Geometry: final body of the model. Coordinates: model frame, mm. Face numbers are marked on the shaded views. Coordinates: 2 decimals unless noted, no trailing zeros. Loops run counter-clockwise (first coordinate to the right, second up) from the corner with the lowest first, then second, coordinate; pieces in that order, holes last. Notation, with made-up numbers: (59, 29.25) -> (64, 29.25) arc R31 ccw to (64, 54.25) -> close; hole circle Ø3 at (-28.5, -8.75). An arc over 180 degrees is marked (long way). One line per item, written item: value. Start each with the question number.
from build123d import *

# Parameters (mm, degrees)
SKETCH1_W           = 118
SKETCH1_H           = 70
BOSS_EXTRUDE1_DEPTH = 36
FILLET1_R           = 2
SKETCH2_W           = 15
SKETCH2_H           = 8
CUT_EXTRUDE1_DEPTH  = 10


with BuildPart() as part:
    # Sketch1 → Boss-Extrude1 (new body)
    with BuildSketch(Plane(origin=(0, 0, 0), x_dir=(1, 0, 0), z_dir=(0, 1, 0))):
        Rectangle(SKETCH1_W, SKETCH1_H)
    extrude(amount=BOSS_EXTRUDE1_DEPTH)

    # Fillet1
    fillet1_edges = [part.edges().sort_by_distance(p)[0] for p in [
        (-59, 36, 0),
        (0, 36, 35),
        (59, 36, 0),
        (0, 0, 35),
        (-59, 0, 0),
        (0, 0, -35),
        (59, 0, 0),
        (59, 18, 35),
        (-59, 18, 35),
        (-59, 18, -35),
        (59, 18, -35),
        (0, 36, -35),
    ]]
    fillet(fillet1_edges, radius=FILLET1_R)

    # Sketch2 → Cut-Extrude1 (cut)
    with BuildSketch(Plane.ZY.offset(59)):
        with Locations((-22.5, 18)):
            Rectangle(SKETCH2_W, SKETCH2_H)
        with Locations((23.5, 18)):
            Rectangle(SKETCH2_W, SKETCH2_H)
        with BuildLine():
            Line((-3, 20.5), (2, 20.5))
            ThreePointArc((2, 20.5), (4.5, 18), (2, 15.5))
            Line((2, 15.5), (-3, 15.5))
            ThreePointArc((-3, 15.5), (-5.5, 18), (-3, 20.5))
        make_face()
    extrude(amount=-CUT_EXTRUDE1_DEPTH, mode=Mode.SUBTRACT)


solid = part.part
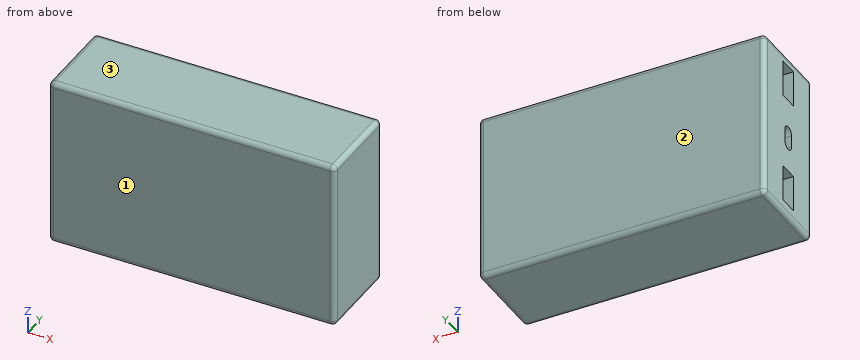
1. Section A-A on z = -21.5. Return the cut outline in (x, y), plus the area to 3 significant figures.
2. Pin query (flat end, axial travel): pin 1 Ø1.5 at (y, z) = (19, -2) entering from -X. Return the tip coordinate at first contact, or that it passes through.
3. Section B-B on y = 18. Return the cut outline in (x, z).
4. Line query: L1, parallel to X at y = 34.5, z = -22.5; L2, parallel to Z at x = -3, y = 34.5. Output: solid intervals per line, ascending. Write a range as [from, to].
5. Draft query along Y for the marked faces 1, 2 and 3. Return one class per face: released by +Y, released by -Y, zero draft, split by the parting line, or undercut.
Checks:
1. outline: (-59, 2) arc R2 ccw to (-57, 0) -> (57, 0) arc R2 ccw to (59, 2) -> (59, 34) arc R2 ccw to (57, 36) -> (-57, 36) arc R2 ccw to (-59, 34) -> (-59, 22) -> (-49, 22) -> (-49, 14) -> (-59, 14) -> close
1. area: 4,160 mm²
2. pin 1: x = -49
3. outline: (-59, -33) arc R2 ccw to (-57, -35) -> (57, -35) arc R2 ccw to (59, -33) -> (59, 33) arc R2 ccw to (57, 35) -> (-57, 35) arc R2 ccw to (-59, 33) -> (-59, 31) -> (-49, 31) -> (-49, 16) -> (-59, 16) -> (-59, 4.5) -> (-49, 4.5) -> (-49, -5.5) -> (-59, -5.5) -> (-59, -15) -> (-49, -15) -> (-49, -30) -> (-59, -30) -> close
4. L1: [-58.94, 58.94]
4. L2: [-34.94, 34.94]
5. face 1: released by -Y
5. face 2: released by +Y
5. face 3: zero draft
